Autodesk Inventor part; units mm, degrees
ref_plane "YZ Plane" through (0, 0, 0) normal (1, 0, 0) x (0, 1, 0)
ref_plane "XZ Plane" through (0, 0, 0) normal (0, 1, 0) x (-1, 0, 0)
ref_plane "XY Plane" through (0, 0, 0) normal (0, 0, 1) x (1, 0, 0)
sketch "Esboço1" plane through (0, 0, 0) normal (0, 1, 0) x (-1, 0, 0)
  circle A0 centre (0, 0) radius 4
  dimension "d1" = 8
extrude "Extrusão1" add sketch "Esboço1" along normal blind 60
sketch "Esboço4" plane through (0, 60, 0) normal (0, 1, 0) x (1, 0, 0)
  circle A0 centre (0, 0) radius 4
hole "Furo1" at (0, 60, 0) direction (0, -1, 0) diameter 4.134 depth 14.2 tip angle 118
sketch "Esboço5" plane through (0, 0, 0) normal (0, -1, 0) x (1, 0, 0)
  circle A0 centre (0, 0) radius 4
hole "Furo2" at (0, 0, 0) direction (0, 1, 0) diameter 4.134 depth 14.2 tip angle 118
equation "\"Raio_vergadura\" = Espessura"
equation "\"Largura_alívio_de_vergadura\" = Espessura"
equation "\"Profundidade_alívio_de_vergadura\" = 0.5 * Espessura"
equation "\"Tamanho_alívio_de_dobra\" = 4 * Espessura"
equation "\"Remanescente_mínimo\" = 2 * Espessura"
equation "\"Raiodetransição\" = Raio_vergadura"
equation "\"Tamanho_de_raio_de_Jacobi\" = Raio_vergadura"
equation "\"TamanhoFolga\" = Espessura"
properties part number "Suporte da base de apoio" material "Latão, amarelo macio"
Can you work these out from the model? Positions are in its coordinate system, mm. A direction names the side the tool comes from. Round coordinates to 2 decimals unless told otherwise and drop trailing zeros. Write each loop counter-clockwise with the first axis right and the second up, starting at its lowest first coordinate (ties: lowest second). Pieces come first, ordered by that corner, then holes. Notation, with made-up numbers: (46.5, 36) -> (82.5, 36) arc R21 ccw to (82.5, 57) -> close; hole circle Ø9 at (21, 86.5). An arc over 180 degrees is marked (long way). Use one line per item in the form item = value. Start each with the question number.
Q1. Imagine slicing it at B-B (x = 3). Please give me the cut outline in (y, z), then the cut area to 3 significant figures.
Q2. Imagine slicing it at A-A (y = 46.5). Please give me the cut outline in (x, z), then the cut area to 3 significant figures.
Q3. Which directions (+Z, -Z, +X, -X, +Y, -Y) give clear straight access to the entire face, cutting with the end or side of a thin tool? Please do faces 1 (the face through (-2, 60, -2)), 2 (the face through (1.26, 7.2, 1.64)).
Q4. I'm going to push flat-ended pins straight in: P1, Ø4, axis at x = -2.5, y = 15.5, coming from the -Z side; P2, Ø3.5, axis at x = 0, z = 0, coming from the -Y side; P3, Ø2.5, axis at x = 0, z = 0, coming from the -Y side. Where does each tip first touch, or does it pass through?
Q5. We'd pull the mould along Z, two halves only. Please class faces 3 (the face through (-2, 0, -2)), 4 (the face through (1.26, 52.8, -1.64)), 5 (the face through (0.867, 29.58, 3.905)): +Z half, -Z half, draft (parallel to the pull), parting line (faces both ways), or undercut.
Q6. If I drill on probe 1 along Z at (x, y) = (0, 7); probe 2 along X at (y, z) = (57, -0.5); probe 3 along Z at (x, y) = (-0.75, 7.5), over which ranges is the centre line in solid material (lowest first)? Write a range as [from, to].
Worked out:
q1.outline = (0, -2.65) -> (60, -2.65) -> (60, 2.65) -> (0, 2.65) -> close
q1.area = 317 mm^2
q2.outline = circle Ø8 at (0, 0); hole circle Ø4.13 at (0, 0)
q2.area = 36.8 mm^2
q3.face_1 = +Z, -Z, +X, -X, +Y
q3.face_2 = -Y
q4.P1 = -3.97
q4.P2 = 14.39
q4.P3 = 14.69
q5.face_3 = draft
q5.face_4 = undercut
q5.face_5 = parting line
q6.probe_1 = [-4, -2.07], [2.07, 4]
q6.probe_2 = [-3.97, -2.01], [2.01, 3.97]
q6.probe_3 = [-3.93, -1.93], [1.93, 3.93]
